Autodesk Inventor part; units mm, degrees
ref_plane "YZ Plane" through (0, 0, 0) normal (1, 0, 0) x (0, 1, 0)
ref_plane "XZ Plane" through (0, 0, 0) normal (0, 1, 0) x (-1, 0, 0)
ref_plane "XY Plane" through (0, 0, 0) normal (0, 0, 1) x (1, 0, 0)
sketch "Sketch1" plane through (0, 0, 0) normal (1, 0, 0) x (0, 1, 0)
  line L0 (85, 22.5) -> (-85, 22.5)
  line L1 (-85, 22.5) -> (-85, -22.5)
  line L2 (-85, -22.5) -> (85, -22.5)
  line L3 (85, -22.5) -> (85, 22.5)
  point P0 (0, 0)
  point P1 (85, 0)
  point P2 (0, 22.5)
  dimension "d0" = 170
  dimension "d1" = 45
extrude "Extrusion1" add sketch "Sketch1" along normal mid plane 10
sketch "Sketch2" plane through (5, 0, 0) normal (1, 0, 0) x (0, 0, -1)
  line L0 (-13.5, -62.5) -> (13.5, -62.5) construction
  line L1 (-22.5, -85) -> (22.5, -85) construction
  point P0 (0, 0)
  point P1 (0, -62.5)
  dimension "d4" = 27
  dimension "d5" = 22.5
hole "BCA M8" at (5, -62.5, 13.5) at (5, -62.5, -13.5) direction (-1, 0, 0) diameter 8 end through all
sketch "Sketch3" plane through (5, 0, 0) normal (1, 0, 0) x (0, 0, -1)
  line L0 (22.5, 85) -> (-22.5, 85)
  point P0 (0, 0)
  point P1 (0, 62.5)
  dimension "d13" = 22.5
hole "Hole2" at (5, 62.5, 0) direction (-1, 0, 0) diameter 8 end through all
properties part number "Sujetador prensa Trigger"
For this review, take the finished solid that the model builds, in its own axes (mm). Coordinates: 2 decimals unless noted, no trailing zeros. Write each loop counter-clockwise with the first axis right and the second up, starting at its lowest first coordinate (ties: lowest second). Pieces come first, ordered by that corner, then holes. Notation, with made-up numbers: (-17.5, -40) - (0.5, -40) arc R15 cw to (0.5, -22) - close; hole circle Ø11 at (-9.75, -28.5). An arc over 180 degrees is marked (long way). Put each result on its own line as item: value.
1. For pin 1 (10.5 mm diameter, centred on y = -62.5, z = 13.5, fed in from +X), flat-tipped, find the tip position at first contact; note if it passes through.
Values found:
pin 1: x = 5
2. Add section A-A, the plane y = 62.5. Give the boundary of the cut face in (x, z), then the cut area to 3 significant figures.
Values found:
outline: (-5, -22.5) - (5, -22.5) - (5, -4) - (-5, -4) - close; (-5, 4) - (5, 4) - (5, 22.5) - (-5, 22.5) - close
area: 370 mm²
3. Mouldability with a two-part tool opening along Z and no side actions: class faces 1 (the cylindrical face through (-0.07, -58.595, 14.367)), 2 (the cylindrical face through (-0.07, 66.405, 0.867)), 3 (the flat face through (0, 1, 22.5)), 4 (the flat face through (0, -85, 0)) as released by +Z, released by -Z, zero draft, split by the parting line, or undercut.
Values found:
face 1: undercut
face 2: undercut
face 3: released by +Z
face 4: zero draft
4. Wall thickness on probe 1 along Z at (x, y) = (0.25, -63); probe 2 along Z at (x, y) = (2.75, 62.5); probe 3 along Y at (x, z) = (0.25, 13.5): over which ranges is each line inside the solid? List them lowest first.
Values found:
probe 1: -22.5 to -17.47, -9.53 to 9.53, 17.47 to 22.5
probe 2: -22.5 to -4, 4 to 22.5
probe 3: -85 to -66.5, -58.5 to 85
5. Add section C-C, the plane x = 1.25. Give the boundary of the cut face in (y, z), then the cut area to 3 significant figures.
Values found:
outline: (-85, -22.5) - (85, -22.5) - (85, 22.5) - (-85, 22.5) - close; hole circle Ø8 at (-62.5, -13.5); hole circle Ø8 at (-62.5, 13.5); hole circle Ø8 at (62.5, 0)
area: 7,500 mm²
6. Add section D-D, the plane y = -62.5. Give the boundary of the cut face in (x, z).
Values found:
outline: (-5, -22.5) - (5, -22.5) - (5, -17.5) - (-5, -17.5) - close; (-5, -9.5) - (5, -9.5) - (5, 9.5) - (-5, 9.5) - close; (-5, 17.5) - (5, 17.5) - (5, 22.5) - (-5, 22.5) - close
7. Add section B-B, the plane z = 0. Give the boundary of the cut face in (x, y).
Values found:
outline: (-5, -85) - (5, -85) - (5, 58.5) - (-5, 58.5) - close; (-5, 66.5) - (5, 66.5) - (5, 85) - (-5, 85) - close
